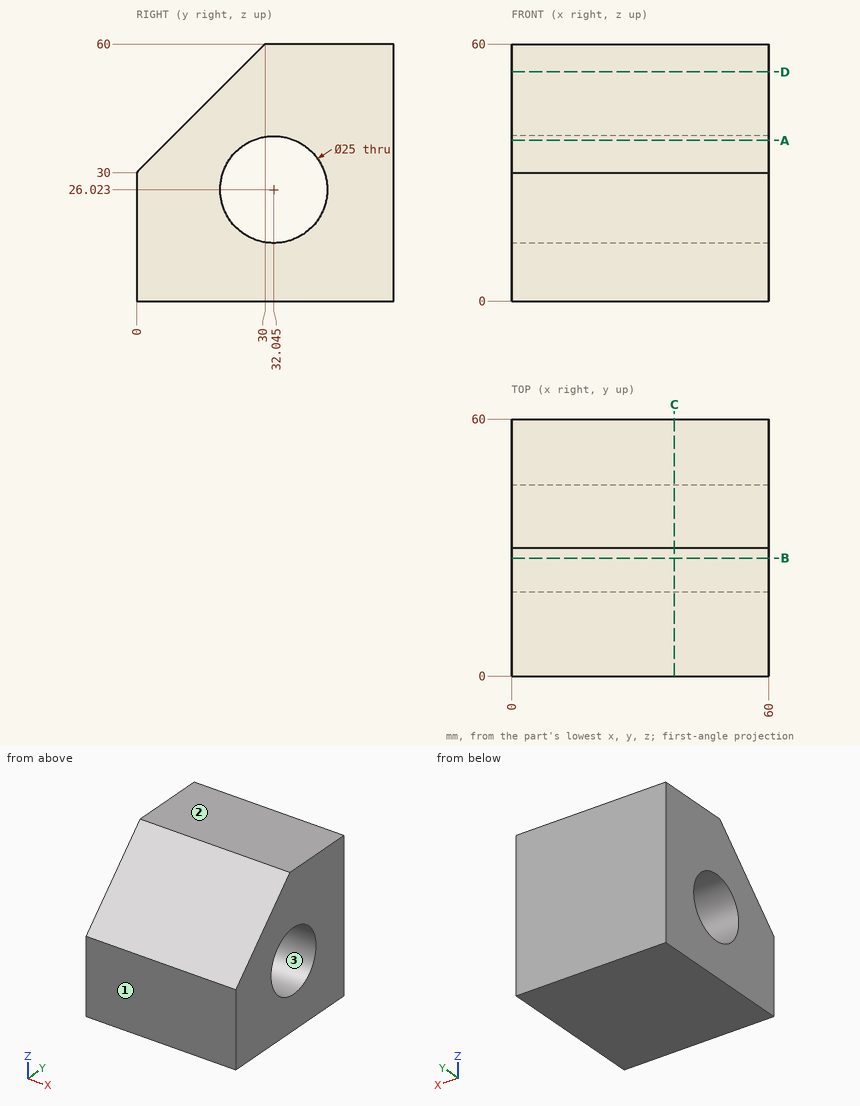
Here's the drawing with two shaded views (mm, measured from the low corner). I have some questions. Round coordinates to 2 decimals unless told otherwise and drop trailing zeros. Write each loop counter-clockwise with the first axis right and the second up, starting at its lowest first coordinate (ties: lowest second). Pieces come first, ordered by that corner, then holes. Notation, with made-up numbers: M 24,38.25 L 61,38.25 A18 ccw 61,63.25 Z; hole C -36,-21 d10. An arc over 180 degrees is marked long. Use CSV: the item, a comma, the result in double quotes.
(1) I need wall thicknesses on line 1 along Z through (x, y) = (28, 43) (1 decimal); line 2 along Y through (x, z) = (21.5, 32) (1 decimal); line 3 along Y through (x, z) = (23.5, 34). Which ranges of each line are inside material? Lowest first, please.
Check values:
line 1,"0 to 20, 32 to 60"
line 2,"2 to 21.1, 43 to 60"
line 3,"4 to 22.42, 41.67 to 60"
(2) Imagine slicing it at C-C (x = 38). Write out the boundary of the cut face in (y, z) (1 decimal), plus the area to 3 significant figures.
Check values:
outline,"M 0,0 L 60,0 L 60,60 L 30,60 L 0,30 Z; hole C 32,26 d25"
area,"2,660 mm^2"
(3) Imagine slicing it at A-A (z = 37.5). Write out the boundary of the cut face in (x, y).
Check values:
outline,"M 0,7.5 L 60,7.5 L 60,27.09 L 0,27.09 Z; M 0,37 L 60,37 L 60,60 L 0,60 Z"
(4) I'm going to push flat-ended pins straight in: pin 1 (10 mm diameter, centred on x = 44.5, z = 36, fed in from -Y); pin 2 (8 mm diameter, centred on y = 37, z = 36.5, fed in from +X); pin 3 (1 mm diameter, centred on x = 44, z = 46, fed in from -Y); pin 4 (2 mm diameter, centred on x = 29, z = 42.5, fed in from -Y). Where does each tip first touch, or does it pass through?
Check values:
pin 1,"y = 1"
pin 2,"x = 60"
pin 3,"y = 15.5"
pin 4,"y = 11.5"
(5) Imagine slicing it at D-D (z = 53.5). Write out the boundary of the cut face in (x, y).
Check values:
outline,"M 0,23.5 L 60,23.5 L 60,60 L 0,60 Z"
(6) Imagine slicing it at B-B (y = 27.5). Write out the boundary of the cut face in (x, z).
Check values:
outline,"M 0,0 L 60,0 L 60,14.38 L 0,14.38 Z; M 0,37.67 L 60,37.67 L 60,57.5 L 0,57.5 Z"
(7) We'd pull the mould along Y, two halves only. Please class the marked faces 1, 2 and 3: +Y half, -Y half, draft (parallel to the pull), parting line (faces both ways), or undercut.
Check values:
face 1,"-Y half"
face 2,"draft"
face 3,"undercut"
